from build123d import *

# Parameters (mm, degrees)
F_5_8_18_TAPPED_HOLE2_D     = 14.68374
F_5_8_18_TAPPED_HOLE2_DEPTH = 38.862
F_5_8_18_TAPPED_HOLE2_TIP   = 4.411440553


with BuildPart() as part:
    # Sketch4 → Revolve1 (revolve)
    with BuildSketch(Plane.XY, mode=Mode.PRIVATE) as revolve1_sk:
        with BuildLine():
            Line((20.32, 59.765541746), (20.32, 53.415541746))
            ThreePointArc((20.32, 53.415541746), (47.050029224, 32.440981027), (57.15, 0))
            Line((57.15, 0), (57.15, -187.884458254))
            ThreePointArc((57.15, -187.884458254), (40.411152545, -228.295610799), (0, -245.034458254))
            Line((0, -245.034458254), (0, -238.684458254))
            ThreePointArc((0, -238.684458254), (35.921024484, -223.805482738), (50.8, -187.884458254))
            Line((50.8, -187.884458254), (50.8, 0))
            ThreePointArc((50.8, 0), (40.560547334, 30.58565023), (13.97, 48.841366688))
            ThreePointArc((13.97, 48.841366688), (8.309203928, 50.115837118), (2.54, 50.736460263))
            Line((2.54, 50.736460263), (2.54, 59.765541746))
            Line((2.54, 59.765541746), (13.97, 59.765541746))
            Line((13.97, 59.765541746), (20.32, 59.765541746))
        make_face()
    revolve(revolve1_sk.sketch.rotate(Axis((0, 80.447885323, 0), (0, -1, 0)), 180), axis=Axis((0, 80.447885323, 0), (0, -1, 0)))

    # 5_8-18 Tapped Hole2
    with Locations(Plane(origin=(0, 59.765541746, 0), x_dir=(1, 0, 0), z_dir=(0, 1, 0))):
        with Locations((0, 0)):
            Hole(F_5_8_18_TAPPED_HOLE2_D / 2, depth=F_5_8_18_TAPPED_HOLE2_DEPTH)
            with Locations((0, 0, -(F_5_8_18_TAPPED_HOLE2_DEPTH + F_5_8_18_TAPPED_HOLE2_TIP / 2))):  # 118° drill point
                Cone(0, F_5_8_18_TAPPED_HOLE2_D / 2, F_5_8_18_TAPPED_HOLE2_TIP, mode=Mode.SUBTRACT)


solid = part.part
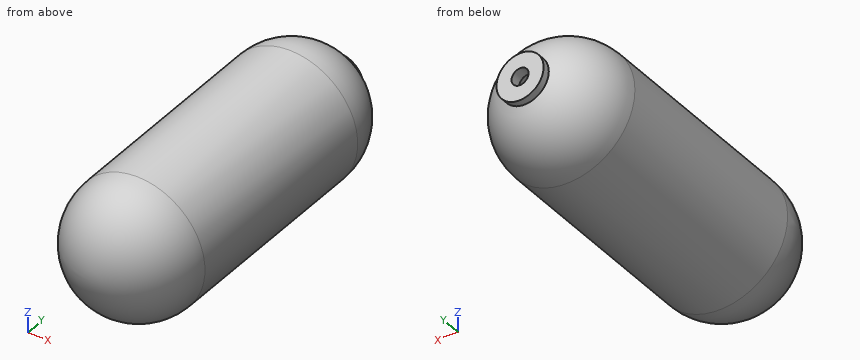
Work out the finished part from the listing and answer in its coordinate system (mm). Give positions to 0.01 mm unless a question says otherwise; leave off trailing zeros. Loops run counter-clockwise (first coordinate to the right, second up) from the corner with the lowest first, then second, coordinate; pieces in that order, holes last. Notation, with made-up numbers: (67, -23.5) -> (99, -23.5) arc R12 ccw to (99, -15.5) -> close; hole circle Ø1 at (76.5, 80.5). An arc over 180 degrees is marked (long way). Use a Markdown table: item, result. Add a question column.
1. Section B-B on x = 42 is taken. Determine the outline of the cut face in (y, z), and give its area (3 significant figures).
2. Find the intervals of material crossed by probe 1 along Z at (x, y) = (0, 56); probe 2 along Y at (x, z) = (-34.5, -12.5); probe 3 along Z at (x, y) = (30, -171.5), in increasing order.
3. Section C-C on y = -34.5 is taken. Determine the outline of the cut face in (x, z), and give its area (3 significant figures).
4. Section A-A on z = 0 is taken. Determine the outline of the cut face in (x, y), and give its area (3 significant figures).
5. Flat-ended cylindrical pins translate along their axes: pin 1 Ø3 at (y, z) = (-36.5, -26) entering from +X; pin 2 Ø10 at (x, y) = (45.5, -57.5) entering from -Z; pin 3 Ø6 at (y, z) = (-74, 37.5) entering from +X. Find the tip coordinate at first contact, or state that the pin passes through.
6. Section D-D on x = 0 is taken. Determine the outline of the cut face in (y, z).
Results below:
| question | item | result |
|---|---|---|
| 1 | outline | (-187.88, -38.76) -> (0, -38.76) arc R38.76 ccw to (0, 38.76) -> (-187.88, 38.76) arc R38.76 ccw to start; hole (-187.88, -28.58) -> (0, -28.58) arc R28.58 ccw to (0, 28.58) -> (-187.88, 28.58) arc R28.58 ccw to start |
| 1 | area | 5,980 mm^2 |
| 2 | probe 1 | z = -20.32 to -7.34, 7.34 to 20.32 |
| 2 | probe 2 | y = -231.7 to -223.01, 35.13 to 43.81 |
| 2 | probe 3 | z = -48.64 to -41, 41 to 48.64 |
| 3 | outline | circle Ø114.3 at (0, 0); hole circle Ø101.6 at (0, 0) |
| 3 | area | 2,150 mm^2 |
| 4 | outline | (-57.15, -187.88) arc R57.15 ccw to (57.15, -187.88) -> (57.15, 0) arc R57.15 ccw to (20.32, 53.42) -> (20.32, 59.77) -> (7.34, 59.77) -> (7.34, 50.27) arc R50.8 cw to (50.8, 0) -> (50.8, -187.88) arc R50.8 cw to (-50.8, -187.88) -> (-50.8, 0) arc R50.8 cw to (-7.34, 50.27) -> (-7.34, 59.77) -> (-20.32, 59.77) -> (-20.32, 53.42) arc R57.15 ccw to (-57.15, 0) -> close |
| 4 | area | 4,560 mm^2 |
| 5 | pin 1 | stops at x = 51.63 |
| 5 | pin 2 | stops at z = -40.32 |
| 5 | pin 3 | stops at x = 45.56 |
| 6 | outline | (-187.88, -57.15) -> (0, -57.15) arc R57.15 ccw to (53.42, -20.32) -> (59.77, -20.32) -> (59.77, -7.34) -> (50.27, -7.34) arc R50.8 cw to (0, -50.8) -> (-187.88, -50.8) arc R50.8 cw to (-187.88, 50.8) -> (0, 50.8) arc R50.8 cw to (50.27, 7.34) -> (59.77, 7.34) -> (59.77, 20.32) -> (53.42, 20.32) arc R57.15 ccw to (0, 57.15) -> (-187.88, 57.15) arc R57.15 ccw to start |
